For this review, take the finished solid that the model builds, in its own axes (mm). A direction names the side the tool comes from. Round coordinates to 2 decimals unless told otherwise and drop trailing zeros. Write each loop counter-clockwise with the first axis right and the second up, starting at its lowest first coordinate (ties: lowest second). Pieces come first, ordered by that corner, then holes. Notation, with made-up numbers: M 24,2 L 42,2 A20 cw 42,40 Z; hole C 9,78 d8. An arc over 180 degrees is marked long. Answer in a Markdown table with one row per item.
```python
from build123d import *

# Parameters (mm, degrees)
SKETCH2_R           = 52.5
SKETCH2_R_2         = 4.1
BOSS_EXTRUDE1_DEPTH = 3.5
SKETCH3_R           = 20.207259422
CUT_EXTRUDE1_DEPTH  = 11.8
BOSS_EXTRUDE2_DEPTH = 3.5
SKETCH5_R           = 7.781762147
BOSS_EXTRUDE3_DEPTH = 11.8


with BuildPart() as part:
    # Sketch2 → Boss-Extrude1 (new body)
    with BuildSketch(Plane.XY):
        Circle(SKETCH2_R)
        with Locations((0, 44)):
            Circle(SKETCH2_R_2, mode=Mode.SUBTRACT)
        with Locations((38.105117767, -22)):
            Circle(SKETCH2_R_2, mode=Mode.SUBTRACT)
        with Locations((-38.105117767, -22)):
            Circle(SKETCH2_R_2, mode=Mode.SUBTRACT)
        Polygon((-17.5, 10.103629711), (0, 20.207259422), (17.5, 10.103629711), (17.5, -10.103629711), (0, -20.207259422), (-17.5, -10.103629711), align=None, mode=Mode.SUBTRACT)
    extrude(amount=BOSS_EXTRUDE1_DEPTH)

    # Sketch3 → Cut-Extrude1 (cut)
    with BuildSketch(Plane(origin=(0, 0, 0), x_dir=(-1, 0, 0), z_dir=(0, 0, -1))):
        Circle(SKETCH3_R)
    extrude(amount=-CUT_EXTRUDE1_DEPTH, mode=Mode.SUBTRACT)

    # Sketch4 → Boss-Extrude2 (add)
    with BuildSketch(Plane(origin=(0, 0, 0), x_dir=(-1, 0, 0), z_dir=(0, 0, -1))):
        with BuildLine():
            Line((2, 9.80418615), (2, 34.404657721))
            Line((2, 34.404657721), (-2, 34.404657721))
            Line((-2, 34.404657721), (-2, 9.80418615))
            Line((-2, 9.80418615), (-1.999978972, 9.598028452))
            ThreePointArc((-1.999978972, 9.598028452), (-6.932952502, 6.932260502), (-9.598228039, 1.999020905))
            Line((-9.598228039, 1.999020905), (-9.80318615, 1.999))
            Line((-9.80318615, 1.999), (-34.403657721, 1.999))
            Line((-34.403657721, 1.999), (-34.403657721, -2.001))
            Line((-34.403657721, -2.001), (-9.80318615, -2.001))
            Line((-9.80318615, -2.001), (-9.597820007, -2.000979053))
            ThreePointArc((-9.597820007, -2.000979053), (-6.931538141, -6.933674715), (-1.998020986, -9.598436237))
            Line((-1.998020986, -9.598436237), (-1.998, -9.80418615))
            Line((-1.998, -9.80418615), (-1.998, -34.404657721))
            Line((-1.998, -34.404657721), (2.002, -34.404657721))
            Line((2.002, -34.404657721), (2.002, -9.80418615))
            Line((2.002, -9.80418615), (2.00197893, -9.597611496))
            ThreePointArc((2.00197893, -9.597611496), (6.93367465, -6.931538207), (9.598227996, -1.999021109))
            Line((9.598227996, -1.999021109), (9.80518615, -1.999))
            Line((9.80518615, -1.999), (34.405657721, -1.999))
            Line((34.405657721, -1.999), (34.405657721, 2.001))
            Line((34.405657721, 2.001), (9.80518615, 2.001))
            Line((9.80518615, 2.001), (9.59782005, 2.000978849))
            ThreePointArc((9.59782005, 2.000978849), (6.932260583, 6.93295242), (2.000021028, 9.598019689))
            Line((2.000021028, 9.598019689), (2, 9.80418615))
        make_face()
    extrude(amount=-BOSS_EXTRUDE2_DEPTH)

    # Sketch5 → Boss-Extrude3 (add)
    with BuildSketch(Plane(origin=(0, 0, 0), x_dir=(-1, 0, 0), z_dir=(0, 0, -1))):
        with Locations(Location((0, 0, 0), (0, 0, 180))):
            Circle(SKETCH5_R)
        with BuildLine():
            Line((-3.424908758, 2.6), (3.424908758, 2.6))
            ThreePointArc((3.424908758, 2.6), (0, -4.3), (-3.424908758, 2.6))
        make_face(mode=Mode.SUBTRACT)
    extrude(amount=BOSS_EXTRUDE3_DEPTH)


solid = part.part
```
Q1. Take a section at D-D (z = -9.25). State the section outline as (x, y) points.
Found:
| item | result |
|---|---|
| outline | C 0,0 d15.56; hole M -3.42,2.6 A4.3 ccw long 3.42,2.6 Z |
Q2. For probe 1 along Y at (x, z) = (0, -5.5); probe 2 along Y at (x, z) = (0, 2.65); probe 3 along Y at (x, z) = (7, 2.25), list the stretches that pass through material, from the lowest coordinate up.
Found:
| item | result |
|---|---|
| probe 1 | -7.78 to -4.3, 2.6 to 7.78 |
| probe 2 | -52.5 to 39.9, 48.1 to 52.5 |
| probe 3 | -52.03 to -18.96, -6.86 to 6.86, 18.96 to 52.03 |
Q3. Mouldability with a two-part tool opening along Y and no side actions: class faces 1 (the face through (4.183, -6.562, -5.817)), 2 (the face through (-14.425, 14.151, 1.726)), 3 (the face through (1, 1, 3.5)) as +Y half, -Y half, draft (parallel to the pull), parting line (faces both ways), or undercut.
Found:
| item | result |
|---|---|
| face 1 | parting line |
| face 2 | undercut |
| face 3 | draft |
Q4. Insertion check: P1, Ø4, axis at y = -17, z = 2.5, coming from the +X side; P2, Ø3, axis at y = -17.5, z = 2.5, coming from the -X side; P3, Ø10, axis at x = -42, y = -11, coming from the -Z side. Each pin has a flat end and moves straight along its axis. Give the tip position at first contact, or say it passes through.
Found:
| item | result |
|---|---|
| P1 | x = 50.31 |
| P2 | x = -50 |
| P3 | z = 0 |
Q5. Machinability: for faces 4 (the face through (6.988, -6.877, 1.726)), 5 (the face through (0, -1, 0)), 6 (the face through (0, 3, -11.8)), which of the approach directions +Z, -Z, +X, -X, +Y, -Y give a long, thin tool a straight path to every point of the face, cutting with its end or side? Answer none if there is none.
Found:
| item | result |
|---|---|
| face 4 | +Z, -Z |
| face 5 | -Z |
| face 6 | -Z, +X, -X, +Y, -Y |
Q6. Take a section at B-B (y = 44). State the section outline as (x, z) points, then the cut area to 3 significant figures.
Found:
| item | result |
|---|---|
| outline | M -28.64,0 L -4.1,0 L -4.1,3.5 L -28.64,3.5 Z; M 4.1,0 L 28.64,0 L 28.64,3.5 L 4.1,3.5 Z |
| area | 172 mm² |
Q7. Take a section at A-A (x = 0). State the section outline as (y, z) points.
Found:
| item | result |
|---|---|
| outline | M -52.5,0 L -7.78,0 L -7.78,-11.8 L -4.3,-11.8 L -4.3,0 L 2.6,0 L 2.6,-11.8 L 7.78,-11.8 L 7.78,0 L 39.9,0 L 39.9,3.5 L -52.5,3.5 Z; M 48.1,0 L 52.5,0 L 52.5,3.5 L 48.1,3.5 Z |
Q8. Take a section at C-C (x = -11). State the section outline as (y, z) points.
Found:
| item | result |
|---|---|
| outline | M -51.33,0 L -16.95,0 L -16.95,3.5 L -51.33,3.5 Z; M -2,0 L 2,0 L 2,3.5 L -2,3.5 Z; M 16.95,0 L 51.33,0 L 51.33,3.5 L 16.95,3.5 Z |
